Could you check a few things on this model? Use its own coordinates, in mm. A direction names the side the tool comes from. Give positions to 0.01 mm unless a question says otherwise; leave off trailing zeros. Order: outer loops, then holes, each group sorted by start corner. A loop starts at its lowest first (then second) coordinate and runs counter-clockwise, first axis right, second up. Notation, with made-up numbers: (88, 47) -> (95, 47) arc R6 ccw to (95, 57) -> close; hole circle Ø1 at (23, -5). An arc over 180 degrees is marked (long way). One line per item, written item: value.
```python
from build123d import *

# Parameters (mm, degrees)
SPIGOT_START          = 105
SKETCH1_W             = 12.1
SKETCH1_H             = 12.1
SPIGOT_DEPTH          = 9
FLANGE_START          = 114
SKETCH2_W             = 24
SKETCH2_H             = 24
FLANGE_DEPTH          = 4
OUTLET_BARB_START     = 118
SKETCH3_R             = 3
OUTLET_BARB_DEPTH     = 9
OUTLET_BARB_TIP_START = 127
SKETCH4_R             = 2.15
OUTLET_BARB_TIP_DEPTH = 7
OUTLET_BORE_START     = 134
SKETCH5_R             = 1.5
OUTLET_BORE_DEPTH     = 29.2
SCREW_HOLES_M3_START  = 113.8
SKETCH6_R             = 1.7
SCREW_HOLES_M3_DEPTH  = 4.4


with BuildPart() as part:
    # Sketch1 → Spigot (new body)
    with BuildSketch(Plane(origin=(0, 0, 0), x_dir=(1, 0, 0), z_dir=(0, 1, 0)).offset(SPIGOT_START)):
        with Locations((14, 0)):
            Rectangle(SKETCH1_W, SKETCH1_H)
    extrude(amount=SPIGOT_DEPTH)

    # Sketch2 → Flange (add)
    with BuildSketch(Plane(origin=(0, 0, 0), x_dir=(1, 0, 0), z_dir=(0, 1, 0)).offset(FLANGE_START)):
        with Locations((14, 0)):
            Rectangle(SKETCH2_W, SKETCH2_H)
    extrude(amount=FLANGE_DEPTH)

    # Sketch3 → Outlet_Barb (add)
    with BuildSketch(Plane(origin=(0, 0, 0), x_dir=(1, 0, 0), z_dir=(0, 1, 0)).offset(OUTLET_BARB_START)):
        with Locations(Location((14, 0, 0), (0, 0, 270))):
            Circle(SKETCH3_R)
    extrude(amount=OUTLET_BARB_DEPTH)

    # Sketch4 → Outlet_Barb_Tip (add)
    with BuildSketch(Plane(origin=(0, 0, 0), x_dir=(1, 0, 0), z_dir=(0, 1, 0)).offset(OUTLET_BARB_TIP_START)):
        with Locations(Location((14, 0, 0), (0, 0, 270))):
            Circle(SKETCH4_R)
    extrude(amount=OUTLET_BARB_TIP_DEPTH)

    # Sketch5 → Outlet_Bore (cut)
    with BuildSketch(Plane(origin=(0, 0, 0), x_dir=(1, 0, 0), z_dir=(0, 1, 0)).offset(OUTLET_BORE_START)):
        with Locations(Location((14, 0, 0), (0, 0, 270))):
            Circle(SKETCH5_R)
    extrude(amount=-OUTLET_BORE_DEPTH, mode=Mode.SUBTRACT)

    # Sketch6 → Screw_Holes_M3 (cut)
    with BuildSketch(Plane(origin=(0, 0, 0), x_dir=(1, 0, 0), z_dir=(0, 1, 0)).offset(SCREW_HOLES_M3_START)):
        with Locations(Location((5.5, 8.5, 0), (0, 0, 270))):
            Circle(SKETCH6_R)
        with Locations(Location((22.5, -8.5, 0), (0, 0, 270))):
            Circle(SKETCH6_R)
    extrude(amount=SCREW_HOLES_M3_DEPTH, mode=Mode.SUBTRACT)


solid = part.part
```
1) Suppose I cut it at B-B, the plane z = 0. Write out the boundary of the cut face in (x, y), then the cut area to 3 significant figures.
Answer below:
outline: (2, 114) -> (7.95, 114) -> (7.95, 105) -> (12.5, 105) -> (12.5, 134) -> (11.85, 134) -> (11.85, 127) -> (11, 127) -> (11, 118) -> (2, 118) -> close; (15.5, 105) -> (20.05, 105) -> (20.05, 114) -> (26, 114) -> (26, 118) -> (17, 118) -> (17, 127) -> (16.15, 127) -> (16.15, 134) -> (15.5, 134) -> close
area: 202 mm2
2) Suppose I cut it at D-D, the plane z = 4.5. Write out the boundary of the cut face in (x, y), then the cut area to 3 significant figures.
Answer below:
outline: (2, 114) -> (7.95, 114) -> (7.95, 105) -> (20.05, 105) -> (20.05, 114) -> (26, 114) -> (26, 118) -> (2, 118) -> close
area: 205 mm2
3) For P1, Ø1, axis at y = 127, z = -2, coming from the +X side; P2, Ø4, axis at x = 8, z = 2, coming from the +Y side; P3, Ø4, axis at x = 22, z = 3.5, coming from the -Y side; P4, Ø2.5, axis at y = 111, z = -1.5, coming from the +X side, each with a flat end and sliding along its axis, tell me the tip position at first contact or that it passes through.
Answer below:
P1: stops at x = 16.6
P2: stops at y = 118
P3: stops at y = 105
P4: stops at x = 20.05
4) Suppose I cut it at C-C, the plane y = 122. Write out the boundary of the cut face in (x, z).
Answer below:
outline: circle Ø6 at (14, 0); hole circle Ø3 at (14, 0)
5) Suppose I cut it at A-A, the plane x = 22.5. Write out the boundary of the cut face in (y, z).
Answer below:
outline: (114, -12) -> (118, -12) -> (118, 6.8) -> (114, 6.8) -> close; (114, 10.2) -> (118, 10.2) -> (118, 12) -> (114, 12) -> close
6) We'd pull the mould along X, two halves only. Please class faces 5 (the flat face through (2, 116, 0)), 6 (the cylindrical face through (3.84, 115.97, -8.87)), 7 (the flat face through (11, 118, -3)): +X half, -X half, draft (parallel to the pull), parting line (faces both ways), or undercut.
Answer below:
face 5: -X half
face 6: undercut
face 7: draft
7) For faces 1 (the flat face through (20.05, 109, 0)), 2 (the flat face through (7.95, 109, 0)), 3 (the flat face through (14, 109, 6.05)), 4 (the cylindrical face through (11.07, 122.44, -0.65)), which set-ups out of +Z, -Z, +X, -X, +Y, -Y let a thin tool reach every point of the face, with its end or its side?
Answer below:
face 1: +Z, -Z, +X, -Y
face 2: +Z, -Z, -X, -Y
face 3: +Z, +X, -X, -Y
face 4: +Y
8) If I drill on line 1 along X through (y, z) = (115.65, -8.5); line 2 along Z through (x, y) = (5.5, 116); line 3 along Z through (x, y) = (22.5, 117.5), over which ranges is the centre line in solid material (lowest first)?
Answer below:
line 1: x = 2 to 3.8, 7.2 to 26
line 2: z = -12 to -10.2, -6.8 to 12
line 3: z = -12 to 6.8, 10.2 to 12
